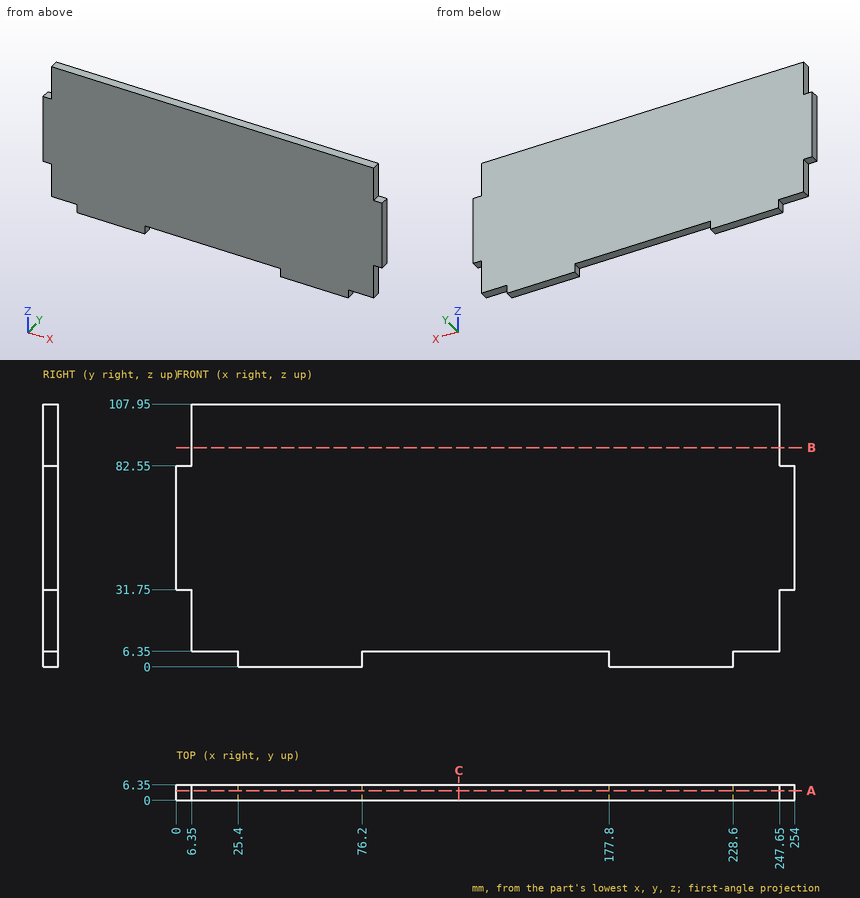
Source: three-view drawing plus pictorial views. Frame: mm from the lowest corner of the part. Give positions to 0.01 mm unless a question says otherwise; leave off trailing zeros. Write each loop counter-clockwise with the first axis right and the second up, starting at its lowest first coordinate (ties: lowest second). Pieces come first, ordered by that corner, then holes. Notation, with made-up numbers: (10.5, -2) - (49.5, -2) arc R15 cw to (49.5, 5) - close; hole circle Ø8 at (7, -26). An arc over 180 degrees is marked (long way). Write item = value, one per line. Start each with the question number.
1. Section query B-B, the plane z = 90. Output: boundary loops of the cut face in (x, y), then the cut area to 3 significant figures.
2. First-contact query: pin 1 Ø3 at (y, z) = (3.5, 4) entering from +X; pin 2 Ø1.9 at (x, y) = (249.5, 2.5) entering from +Z; pin 3 Ø3 at (x, y) = (11.5, 2) entering from -Z. Flat tips, straight axial feed; report the tip coordinate or a pass-through.
3. Ray query, L1, parallel to X at y = 2.75, z = 5.5; L2, parallel to X at y = 2.25, z = 10; L3, parallel to Z at x = 141, y = 2.75. Return the intervals inside material, ascending.
4. Section query C-C, the plane x = 116. Output: boundary loops of the cut face in (y, z), then the cut area to 3 significant figures.
5. Section query A-A, the plane y = 4. Output: boundary loops of the cut face in (x, z).
Check sheet entries:
q1.outline = (6.35, 0) - (247.65, 0) - (247.65, 6.35) - (6.35, 6.35) - close
q1.area = 1,530 mm2
q2.pin_1 = 228.6
q2.pin_2 = 82.55
q2.pin_3 = 6.35
q3.L1 = 25.4 to 76.2, 177.8 to 228.6
q3.L2 = 6.35 to 247.65
q3.L3 = 6.35 to 107.95
q4.outline = (0, 6.35) - (6.35, 6.35) - (6.35, 107.95) - (0, 107.95) - close
q4.area = 645 mm2
q5.outline = (0, 31.75) - (6.35, 31.75) - (6.35, 6.35) - (25.4, 6.35) - (25.4, 0) - (76.2, 0) - (76.2, 6.35) - (177.8, 6.35) - (177.8, 0) - (228.6, 0) - (228.6, 6.35) - (247.65, 6.35) - (247.65, 31.75) - (254, 31.75) - (254, 82.55) - (247.65, 82.55) - (247.65, 107.95) - (6.35, 107.95) - (6.35, 82.55) - (0, 82.55) - close
